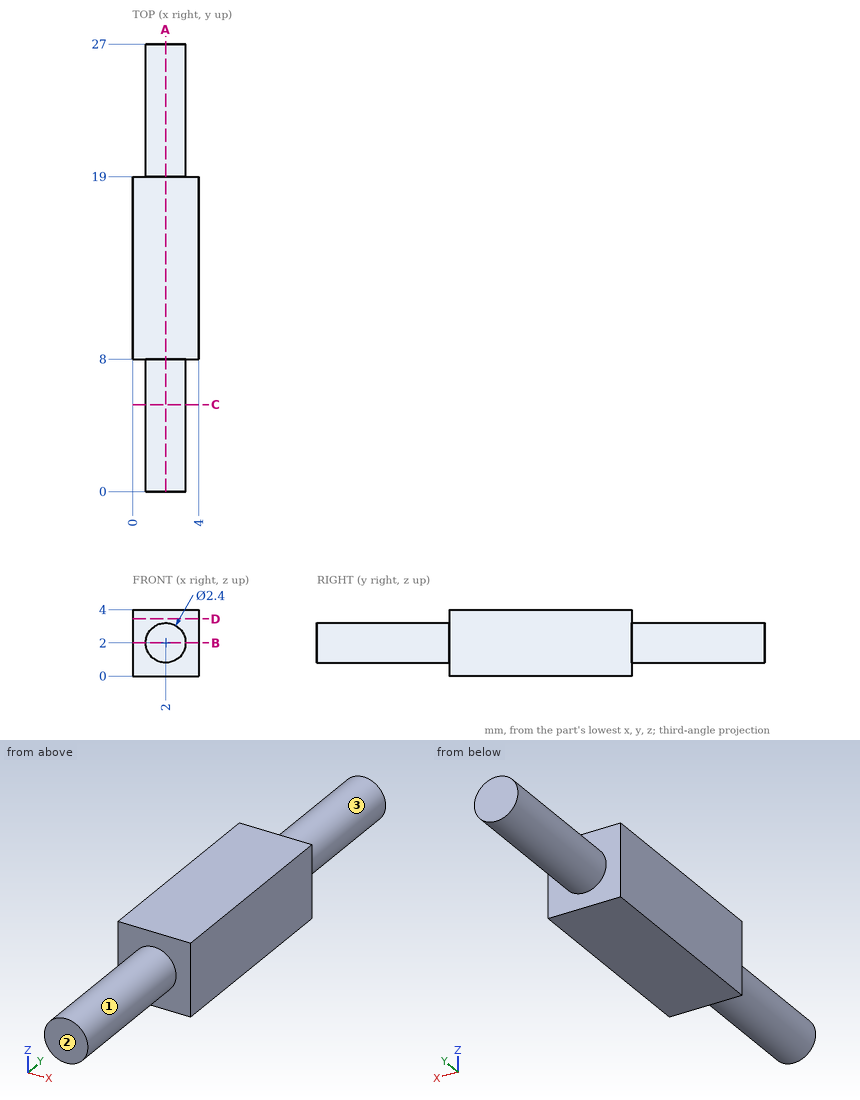
Print and shaded views of the part. All mm, measured from the part's lowest x, y and z. A direction names the side the tool comes from. Coordinates: 2 decimals unless noted, no trailing zeros. Loops run counter-clockwise (first coordinate to the right, second up) from the corner with the lowest first, then second, coordinate; pieces in that order, holes last. Notation, with made-up numbers: (-35, -15) - (-15, -15) arc R28 ccw to (-15, 12) - close; hole circle Ø8 at (28.25, 35.25). An arc over 180 degrees is marked (long way). Write item = value, one per line. Start each with the question number.
Item 1: Saw through at C-C, the plane y = 5.25. List the corners of the cut face in (x, z).
Item 2: Saw through at B-B, the plane z = 2. List the corners of the cut face in (x, y), then the cut area to 3 significant figures.
Item 3: 3-axis set-ups, long thin cutter, end or side, ignore diameter. For the marked faces 1, 2 and 3: which of +Z, -Z, +X, -X, +Y, -Y reach the whole face in a straight line?
Item 4: Saw through at D-D, the plane z = 3.45. List the corners of the cut face in (x, y).
Item 5: Drop flat-ended pins along their axis: pin 1 Ø1.5 at (x, z) = (1, 0.5) entering from +Y; pin 2 Ø1 at (y, z) = (21.5, 2.5) entering from +X. Give the stop position or say it passes through.
Item 6: Wall check: probe 1 along Y at (x, z) = (0.8, 2.3); probe 2 along Z at (x, y) = (2, 6.5); probe 3 along Z at (x, y) = (2.5, 6). Give the ranges that are in metal, low to high. Write a range as [from, to].
Item 7: Saw through at A-A, the plane x = 2. List the corners of the cut face in (y, z), then the cut area to 3 significant figures.
Answers:
q1.outline = circle Ø2.4 at (2, 2)
q2.outline = (0, 8) - (0.8, 8) - (0.8, 0) - (3.2, 0) - (3.2, 8) - (4, 8) - (4, 19) - (3.2, 19) - (3.2, 27) - (0.8, 27) - (0.8, 19) - (0, 19) - close
q2.area = 82.4 mm2
q3.face_1 = -Y
q3.face_2 = +Z, -Z, +X, -X, -Y
q3.face_3 = +Y
q4.outline = (0, 8) - (4, 8) - (4, 19) - (0, 19) - close
q5.pin_1 = 27
q5.pin_2 = 3.2
q6.probe_1 = [8, 19]
q6.probe_2 = [0.8, 3.2]
q6.probe_3 = [0.91, 3.09]
q7.outline = (0, 0.8) - (8, 0.8) - (8, 0) - (19, 0) - (19, 0.8) - (27, 0.8) - (27, 3.2) - (19, 3.2) - (19, 4) - (8, 4) - (8, 3.2) - (0, 3.2) - close
q7.area = 82.4 mm2
